```python
from build123d import *

# Parameters (mm, degrees)
SKETCH_1_W          = 85
SKETCH_1_H          = 47
SKETCH_1_R          = 1.75
SKETCH_1_W_2        = 7
SKETCH_1_H_2        = 3.5
SKETCH_1_H_3        = 3.6
EXTRUDE_1_DEPTH     = 2.5
SKETCH_2_W          = 37
SKETCH_2_H          = 3
EXTRUDE_2_DEPTH     = 4.9
EXTRUDE_START       = 2
SKETCH_3_W          = 37
SKETCH_3_H          = 20.75
SKETCH_3_R          = 1.75
SKETCH_3_W_2        = 7
SKETCH_3_H_2        = 3.5
EXTRUDE_4_DEPTH     = 2
FILLET_1_R          = 3.4
SKETCH_4_W          = 6
SKETCH_4_H          = 3.4
SKETCH_4_W_2        = 5
SKETCH_4_H_2        = 3
SKETCH_4_W_3        = 3
CUT_EXTRUDE_1_DEPTH = 7.4
FILLET_2_R          = 6


with BuildPart() as part:
    # 草图1 → 凸台-拉伸1 (new body)
    with BuildSketch(Plane(origin=(0, 0, 0), x_dir=(1, 0, 0), z_dir=(0, 1, 0))):
        Rectangle(SKETCH_1_W, SKETCH_1_H)
        with Locations(Location((-38.3, -17.5, 0), (0, 0, 270))):
            Circle(SKETCH_1_R, mode=Mode.SUBTRACT)
        with Locations(Location((38.3, -17.5, 0), (0, 0, 270))):
            Circle(SKETCH_1_R, mode=Mode.SUBTRACT)
        with Locations(Location((-38.3, 7.5, 0), (0, 0, 270))):
            Circle(SKETCH_1_R, mode=Mode.SUBTRACT)
        with Locations(Location((38.3, 7.5, 0), (0, 0, 270))):
            Circle(SKETCH_1_R, mode=Mode.SUBTRACT)
        with Locations(Location((-38.3, 17.5, 0), (0, 0, 270))):
            Circle(SKETCH_1_R, mode=Mode.SUBTRACT)
        with Locations(Location((38.3, 17.5, 0), (0, 0, 270))):
            Circle(SKETCH_1_R, mode=Mode.SUBTRACT)
        with Locations((-12.75, -17.5)):
            Rectangle(SKETCH_1_W_2, SKETCH_1_H_2, mode=Mode.SUBTRACT)
        with Locations((12.8, -17.5)):
            Rectangle(SKETCH_1_W_2, SKETCH_1_H_2, mode=Mode.SUBTRACT)
        with Locations((-12.75, 7.5)):
            Rectangle(SKETCH_1_W_2, SKETCH_1_H_3, mode=Mode.SUBTRACT)
        with Locations((12.8, 7.5)):
            Rectangle(SKETCH_1_W_2, SKETCH_1_H_3, mode=Mode.SUBTRACT)
        with Locations((-12.75, 17.5)):
            Rectangle(SKETCH_1_W_2, SKETCH_1_H_2, mode=Mode.SUBTRACT)
        with Locations((12.8, 17.5)):
            Rectangle(SKETCH_1_W_2, SKETCH_1_H_2, mode=Mode.SUBTRACT)
    extrude(amount=EXTRUDE_1_DEPTH)

    # 草图2 → 凸台-拉伸2 (add)
    with BuildSketch(Plane(origin=(0, 0, 0), x_dir=(1, 0, 0), z_dir=(0, 1, 0))):
        with Locations((-24, -4.25)):
            Rectangle(SKETCH_2_W, SKETCH_2_H)
    extrude(amount=-EXTRUDE_2_DEPTH)

    # 草图3 → 凸台-拉伸4 (add)
    with BuildSketch(Plane(origin=(0, -4.9, 0), x_dir=(-1, 0, 0), z_dir=(0, -1, 0)).offset(EXTRUDE_START)):
        with Locations((24, -13.125)):
            Rectangle(SKETCH_3_W, SKETCH_3_H)
        with Locations(Location((38.3, -17.5, 0), (0, 0, 270))):
            Circle(SKETCH_3_R, mode=Mode.SUBTRACT)
        with Locations((12.75, -17.5)):
            Rectangle(SKETCH_3_W_2, SKETCH_3_H_2, mode=Mode.SUBTRACT)
    extrude(amount=-EXTRUDE_4_DEPTH)

    # 圆角1
    fillet_1_edges = [part.edges().sort_by_distance(p)[0] for p in [
        (-5.5, -5.9, 23.5),
        (-42.5, -5.9, 23.5),
        (42.5, 1.25, 23.5),
        (-42.5, 1.25, 23.5),
        (-42.5, 1.25, -23.5),
        (42.5, 1.25, -23.5),
    ]]
    fillet(fillet_1_edges, radius=FILLET_1_R)

    # 草图4 → 切除-拉伸1 (cut)
    with BuildSketch(Plane(origin=(0, -4.9, 0), x_dir=(-1, 0, 0), z_dir=(0, -1, 0))):
        with Locations((26.25, -11.25)):
            Rectangle(SKETCH_4_W, SKETCH_4_H)
        with Locations((13.75, -9.75)):
            Rectangle(SKETCH_4_W_2, SKETCH_4_H_2)
        with Locations((37.75, -9.75)):
            Rectangle(SKETCH_4_W_3, SKETCH_4_H_2)
    extrude(amount=-CUT_EXTRUDE_1_DEPTH, mode=Mode.SUBTRACT)

    # 圆角2
    fillet_2_edges = [part.edges().sort_by_distance(p)[0] for p in [
        (-24, 0, 2.75),
    ]]
    fillet(fillet_2_edges, radius=FILLET_2_R)


solid = part.part
```
CAD build for the part. Positions are in the model's coordinates, mm. A direction names the side the tool comes from. Give positions to 0.01 mm unless a question says otherwise; leave off trailing zeros. Loops run counter-clockwise (first coordinate to the right, second up) from the corner with the lowest first, then second, coordinate; pieces in that order, holes last. Notation, with made-up numbers: (85, 38) - (121, 38) arc R37 ccw to (121, 76) - close; hole circle Ø8 at (88, 17.5). An arc over 180 degrees is marked (long way). Put each result on its own line as item: value.
Q1. Probe line 1 along X through (y, z) = (-5.9, 17.5); line 2 along X through (y, z) = (2, 17.5); line 3 along Z through (x, y) = (-38.3, -5.8). List the from-to ranges inside material, lowest first.
Filled in:
line 1: x = -42.5 to -40.05, -36.55 to -16.25, -9.25 to -5.5
line 2: x = -42.5 to -40.05, -36.55 to -16.25, -9.25 to 9.3, 16.3 to 36.55, 40.05 to 42.5
line 3: z = 2.75 to 15.75, 19.25 to 23.5
Q2. Mould opens along Z. For faces 1 (the face through (41.48, 1.27, -22.53)), 2 (the face through (-38, 1, 8.25)), 3 (the face through (-24, -6, 23.5)) say: pulls with the +Z half, pulls with the -Z half, needs draft (parallel to the pull), parting line crosses it, or undercut.
Filled in:
face 1: pulls with the -Z half
face 2: undercut
face 3: pulls with the +Z half
Q3. Slice it at A-A (x = 38.3). Give the cut face in (y, z), plus the area to 4 significant figures.
Filled in:
outline: (0, -23.5) - (2.5, -23.5) - (2.5, -19.25) - (0, -19.25) - close; (0, -15.75) - (2.5, -15.75) - (2.5, -9.25) - (0, -9.25) - close; (0, -5.75) - (2.5, -5.75) - (2.5, 15.75) - (0, 15.75) - close; (0, 19.25) - (2.5, 19.25) - (2.5, 23.5) - (0, 23.5) - close
area: 91.25 mm²
Q4. Flat gauge pins, fed straight in: pin 1 (1 mm diameter, centred on y = -6.5, z = 17, fed in from +X); pin 2 (6 mm diameter, centred on x = 22, z = 9, fed in from -Y). Where does each tip first touch, or does it go through?
Filled in:
pin 1: stops at x = -5.5
pin 2: stops at y = 0
Q5. Slice it at B-B (x = -38.3). Give the number of separate pieces and of enclosed holes in the cut face, plus the area to 3 significant figures.
Filled in:
separate pieces: 6
enclosed holes: 0
area: 141 mm²
Q6. Slice it at C-C (z = -7.5). Give the cut face in (x, y), plus the area to 3 significant figures.
Filled in:
outline: (-42.5, 0) - (-40.05, 0) - (-40.05, 2.5) - (-42.5, 2.5) - close; (-36.55, 0) - (-16.25, 0) - (-16.25, 2.5) - (-36.55, 2.5) - close; (-9.25, 0) - (9.3, 0) - (9.3, 2.5) - (-9.25, 2.5) - close; (16.3, 0) - (36.55, 0) - (36.55, 2.5) - (16.3, 2.5) - close; (40.05, 0) - (42.5, 0) - (42.5, 2.5) - (40.05, 2.5) - close
area: 160 mm²
Q7. Tool access for faces 4 (the face through (-1, 1, -23.5)), 5 (the face through (-13, 1, -15.75)), 6 (the face through (-11.25, 1, 10)): list every direction of +Z, -Z, +X, -X, +Y, -Y with a clear straight run to the whole face (end or side of a thin tool).
Filled in:
face 4: -Z, +X, -X, +Y, -Y
face 5: +Y, -Y
face 6: +Y
